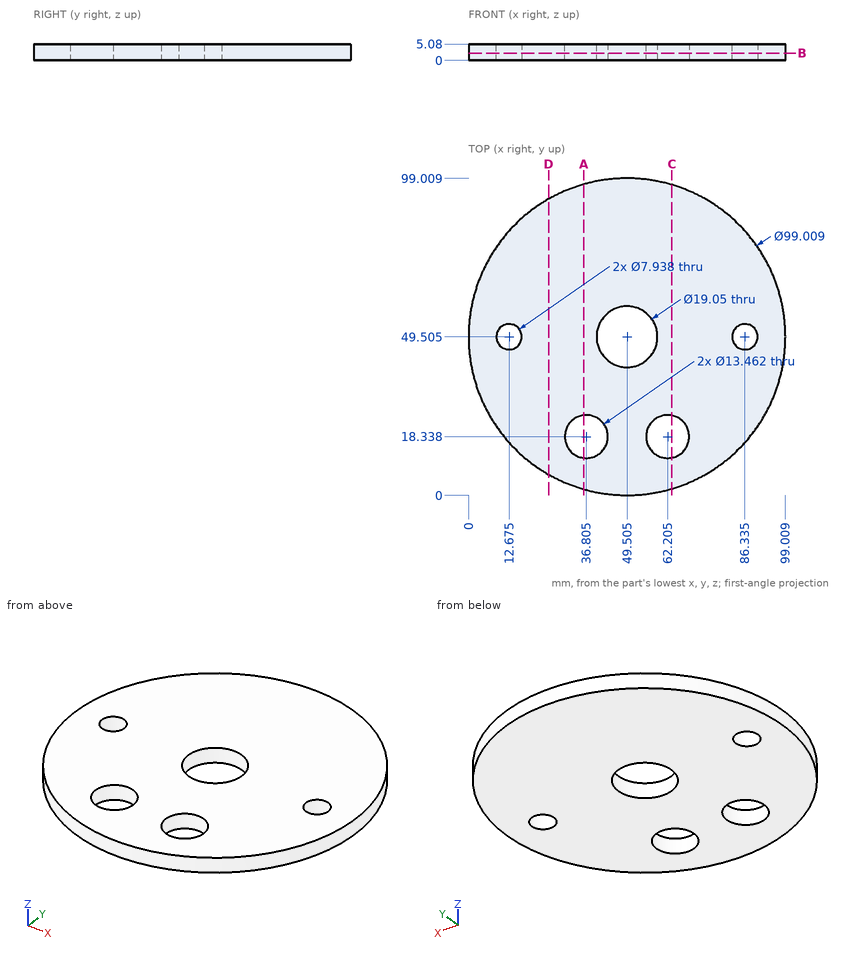
Answer from the drawing. Dimensions are ordinates in mm from the lowest x, y and z of the part. Give positions to 0.01 mm unless a question says otherwise; leave off trailing zeros. Write each loop counter-clockwise with the first axis right and the second up, starting at its lowest first coordinate (ties: lowest second). Pieces come first, ordered by that corner, then holes. Notation, with made-up numbers: (-10.5, 72) - (5.5, 72) arc R8 cw to (5.5, 77) - close; hole circle Ø11 at (-38, 54.5). An arc over 180 degrees is marked (long way). One line per item, written item: value. Start each with the question number.
1. Find section C-C (x = 63.5). Write down the section's boundary in (y, z).
2. Consider probe 1 along X at (y, z) = (19.5, 4.2) (1 decimal); probe 2 along X at (y, z) = (15.5, 2.5) (1 decimal); probe 3 along X at (y, z) = (86.5, 1.4). Determine where each line is inside the solid, lowest interval first.
3. Find section B-B (z = 2.25). State how many separate pieces and enclosed holes the cut face has, then the cut area to 3 significant figures.
4. Given pin 1 (1.5 mm diameter, centred on x = 65.5, z = 1.5, fed in from -Y) (1 decimal); pin 2 (2 mm diameter, centred on y = 16, z = 4, fed in from -X) (1 decimal), each flat-ended and moving along its own axis, determine where each tip first touches the part or whether it passes through.
5. Find section D-D (x = 25). Write down the section's boundary in (y, z).
6. Find section A-A (x = 36). Write down the section's boundary in (y, z) (1 decimal).
Geometry results:
1. outline: (2.02, 0) - (11.73, 0) - (11.73, 5.08) - (2.02, 5.08) - close; (24.94, 0) - (96.99, 0) - (96.99, 5.08) - (24.94, 5.08) - close
2. probe 1: 10.1 to 30.2, 43.4 to 55.6, 68.8 to 88.9
2. probe 2: 13.5 to 30.7, 42.9 to 56.1, 68.3 to 85.5
2. probe 3: 16.61 to 82.4
3. separate pieces: 1
3. enclosed holes: 5
3. area: 7,030 mm2
4. pin 1: y = 2.4
4. pin 2: x = 12.2
5. outline: (6.49, 0) - (92.52, 0) - (92.52, 5.08) - (6.49, 5.08) - close
6. outline: (1.9, 0) - (11.7, 0) - (11.7, 5.1) - (1.9, 5.1) - close; (25, 0) - (97.1, 0) - (97.1, 5.1) - (25, 5.1) - close
